Check sheet for the modelled part. Datum: model origin and axes. Units: mm. Face numbers are marked on the shaded views. A direction names the side the tool comes from. Round coordinates to 2 decimals unless told otherwise and drop trailing zeros. Order: outer loops, then holes, each group sorted by start corner. A loop starts at its lowest first (then second) coordinate and runs counter-clockwise, first axis right, second up. Notation, with made-up numbers: (26.5, 4.25) -> (64.5, 4.25) arc R7 ccw to (64.5, 11.25) -> close; hole circle Ø6 at (-39.5, -8). An arc over 180 degrees is marked (long way). Answer in a Markdown table with one row per item.
```python
from build123d import *

# Parameters (mm, degrees)
F0_R        = 50.8
F1_DEPTH    = 127
F1_FACE_R   = 88.9
F1_FACE_R_2 = 50.8
F2_DEPTH    = 25.4
F3_DEPTH    = 50.8
F4_DEPTH    = 127


with BuildPart() as f1:
    # F0 (on Front) → F1 (new body)
    with BuildSketch(Plane.XZ):
        with BuildLine():
            ThreePointArc((210.733239, 184.80561), (127, 243.84), (43.266761, 184.80561))
            ThreePointArc((43.266761, 184.80561), (111.84538, 67.341213), (215.9, 154.94))
            ThreePointArc((215.9, 154.94), (214.598787, 170.09462), (210.733239, 184.80561))
        make_face()
        with Locations((127, 154.94)):
            Circle(F0_R, mode=Mode.SUBTRACT)
    extrude(amount=F1_DEPTH)

    # F1_face (on face) → F2 (join)
    with BuildSketch(Plane(origin=(127, -127, 154.94), x_dir=(1, 0, 0), z_dir=(0, -1, 0))):
        Circle(F1_FACE_R)
        Circle(F1_FACE_R_2, mode=Mode.SUBTRACT)
    extrude(amount=F2_DEPTH)

    # F0 (on Front) → F3 (join)
    with BuildSketch(Plane.XZ):
        with BuildLine():
            Line((43.266761, 184.80561), (0, 63.5))
            Line((0, 63.5), (254, 63.5))
            Line((254, 63.5), (210.733239, 184.80561))
            ThreePointArc((210.733239, 184.80561), (214.598787, 170.09462), (215.9, 154.94))
            ThreePointArc((215.9, 154.94), (111.84538, 67.341213), (43.266761, 184.80561))
        make_face()
    extrude(amount=F3_DEPTH)

    # F0 (on Front) → F4 (join)
    with BuildSketch(Plane.XZ):
        Polygon((0, 63.5), (0, 0), (83.8623, 0), (45.7623, 38.1), (228.6, 38.1), (190.5, 0), (254, 0), (254, 63.5), align=None)
    extrude(amount=F4_DEPTH)


solid = f1.part
```
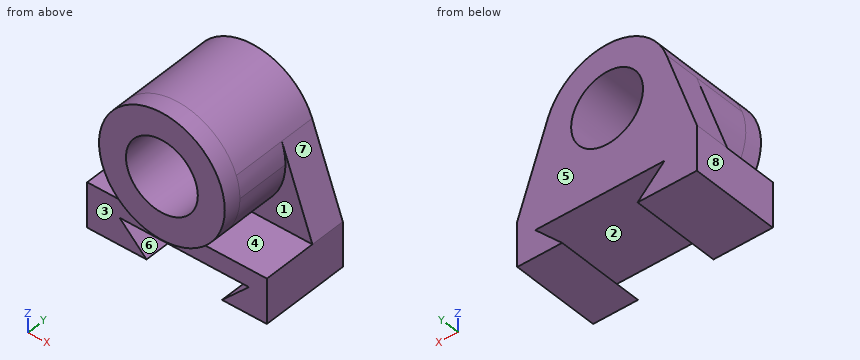
(1) Section check B-B on y = -69. Record the boundary of the cut face in (x, z).
Solutions:
| item | result |
|---|---|
| outline | (0, 0) -> (83.86, 0) -> (45.76, 38.1) -> (228.6, 38.1) -> (190.5, 0) -> (254, 0) -> (254, 63.5) -> (0, 63.5) -> close; (210.73, 184.81) arc R88.9 ccw (long way) to (215.9, 154.94) arc R88.9 ccw to start; hole circle Ø101.6 at (127, 154.94) |
(2) Draft check along X on the marked faces 6, 7 and 8. Enter one of: pulls with the +X half, pulls with the -X half, needs draft (parallel to the pull), parting line crosses it, or undercut.
Solutions:
| item | result |
|---|---|
| face 6 | undercut |
| face 7 | pulls with the +X half |
| face 8 | pulls with the -X half |
(3) Section check A-A on y = -15.5. Record the boundary of the cut face in (x, z).
Solutions:
| item | result |
|---|---|
| outline | (0, 0) -> (83.86, 0) -> (45.76, 38.1) -> (228.6, 38.1) -> (190.5, 0) -> (254, 0) -> (254, 63.5) -> (210.73, 184.81) arc R88.9 ccw to (43.27, 184.81) -> (0, 63.5) -> close; hole circle Ø101.6 at (127, 154.94) |
(4) Section check D-D on z = 166.5. Record the boundary of the cut face in (x, y).
Solutions:
| item | result |
|---|---|
| outline | (36.74, -50.8) -> (38.85, -50.8) -> (38.85, -152.4) -> (77.53, -152.4) -> (77.53, 0) -> (36.74, 0) -> close; (176.47, -152.4) -> (215.15, -152.4) -> (215.15, -50.8) -> (217.26, -50.8) -> (217.26, 0) -> (176.47, 0) -> close |
(5) Scan lines: probe 1 along X at (y, z) = (-68, 154); probe 2 along Z at (x, y) = (163, -90); probe 3 along Y at (x, z) = (63, 44.5). Record each from-to range of solid material in increasing order. Write a range as from..to.
Solutions:
| item | result |
|---|---|
| probe 1 | 38.1..76.21, 177.79..215.9 |
| probe 2 | 38.1..63.5, 73.66..119.1, 190.78..236.22 |
| probe 3 | -127..0 |
(6) Depth check by flat-ended pin: pin 1 Ø6 at (y, z) = (-46.5, 171) entering from -X; pin 2 Ø10 at (x, z) = (136, 109) entering from -Y; pin 3 Ø1.5 at (y, z) = (-135.5, 174) entering from -X; pin 4 Ø19 at (x, z) = (180, 35.5) entering from -Y. Enter the tip coordinate at first touch or a pass-through.
Solutions:
| item | result |
|---|---|
| pin 1 | x = 37.27 |
| pin 2 | y = -152.4 |
| pin 3 | x = 40.01 |
| pin 4 | y = -127 |
(7) Tool access check on the marked faces 1, 2, 3, 4 and 5. Record the directions out of +Z, -Z, +X, -X, +Y, -Y that give a thin tool (end or side, any length) a straight path to the whole face; none if there is none.
Solutions:
| item | result |
|---|---|
| face 1 | -Y |
| face 2 | +Y, -Y |
| face 3 | -Z, +X, -X, -Y |
| face 4 | +X, -X, -Y |
| face 5 | +Z, -Z, +X, -X, +Y |
(8) Section check C-C on x = 127. Record the boundary of the cut face in (y, z).
Solutions:
| item | result |
|---|---|
| outline | (-152.4, 66.04) -> (-50.8, 66.04) -> (-50.8, 63.5) -> (-127, 63.5) -> (-127, 38.1) -> (0, 38.1) -> (0, 104.14) -> (-152.4, 104.14) -> close; (-152.4, 205.74) -> (0, 205.74) -> (0, 243.84) -> (-152.4, 243.84) -> close |
